Source: CAD feature listing. Evaluate the final solid. Frame: model axes, mm. A direction names the side the tool comes from. Round coordinates to 2 decimals unless told otherwise and drop trailing zeros. Write each loop counter-clockwise with the first axis right and the second up, starting at its lowest first coordinate (ties: lowest second). Pieces come first, ordered by that corner, then holes. Notation, with made-up numbers: M 72,-12 L 90,-12 A29 ccw 90,26 Z; hole C 83,-18 d5. An arc over 180 degrees is marked long. Answer in a Markdown table with one row per item. Add a question column.
Item 1: Set-up query: faces 1 (the face through (13.037, 7.419, 3.479)), 2 (the face through (-11.9, 6.97, 0.79)), 3 (the face through (-11.9, 6.97, 6.21)). Return all of +Z, -Z, +X, -X, +Y, -Y with unobstructed straight access to the full face (end or side cutting, diameter ignored); none if empty.
Item 2: Material intervals for probe 1 along Y at (x, z) = (0, 3.25); probe 2 along X at (y, z) = (-9, 5); probe 3 along X at (y, z) = (-23.5, 1), sorted ascending.
Item 3: Contact query for flat-ended pins moving along their axis: pin 1 (13 mm diameter, centred on x = 0, y = 0, fed in from +Z); pin 2 (3 mm diameter, centred on x = 27, z = 4.5, fed in from -Y); pin 3 (10 mm diameter, centred on x = -18.5, y = 7, fed in from -Z); pin 4 (3 mm diameter, centred on x = -28.5, z = 1.5, fed in from +Y). Output: stop coordinate, or through.
Item 4: Cut plane B-B on z = 4. Give the number of separate pieces and of enclosed holes in the cut face, and give its area (3 significant figures).
Item 5: Cut plane A-A on x = 0. Return loops of the section in (y, z), and give its area (3 significant figures).
Item 6: Mould query, pull axis Y, two halves, no side actions, for faces 4 (the face through (-8.69, -6.66, 3.45)), 5 (the face through (0, -14, 6)), 6 (the face through (35.38, -20.96, 6.87)). Classes: released by +Y, released by -Y, zero draft, split by the parting line, or undercut.
from build123d import *

# Parameters (mm, degrees)
F0_R     = 10.95
F1_DEPTH = 7
F2_R     = 2
F3_SIZE  = 2


with BuildPart() as f1:
    # F0 (on Top) → F1 (new body)
    with BuildSketch(Plane.XY):
        with BuildLine():
            ThreePointArc((14.816938, -2.33631), (12.990381, 7.5), (5.385165, 14))
            ThreePointArc((5.385165, 14), (0, 43), (-5.385165, 14))
            ThreePointArc((-5.385165, 14), (-12.990381, 7.5), (-14.816938, -2.33631))
            ThreePointArc((-14.816938, -2.33631), (-37.239092, -21.5), (-9.431773, -11.66369))
            ThreePointArc((-9.431773, -11.66369), (0, -15), (9.431773, -11.66369))
            ThreePointArc((9.431773, -11.66369), (37.239092, -21.5), (14.816938, -2.33631))
        make_face()
        with Locations((-24.248711, -14)):
            Circle(F0_R, mode=Mode.SUBTRACT)
        with Locations((24.248711, -14)):
            Circle(F0_R, mode=Mode.SUBTRACT)
        Circle(F0_R, mode=Mode.SUBTRACT)
        with Locations((0, 28)):
            Circle(F0_R, mode=Mode.SUBTRACT)
    extrude(amount=F1_DEPTH)

    # F2
    f2_edges = [f1.edges().sort_by_distance(p)[0] for p in [
        (-9.431773, -11.66369, 3.5),
        (9.431773, -11.66369, 3.5),
        (14.816938, -2.33631, 3.5),
        (5.385165, 14, 3.5),
        (-5.385165, 14, 3.5),
        (-14.816938, -2.33631, 3.5),
    ]]
    fillet(f2_edges, radius=F2_R)

    # F3
    f3_edges = [f1.edges().sort_by_distance(p)[0] for p in [
        (37.239092, -21.5, 0),
        (37.239092, -21.5, 7),
    ]]
    chamfer(f3_edges, length=F3_SIZE)


solid = f1.part
Results below:
| question | item | result |
|---|---|---|
| 1 | face 1 | +Z, -Z, +X |
| 1 | face 2 | -Z, -X |
| 1 | face 3 | +Z, -X |
| 2 | probe 1 | -15 to -10.95, 10.95 to 17.05, 38.95 to 43 |
| 2 | probe 2 | -38.39 to -33.99, -14.51 to -6.24, 6.24 to 14.51, 33.99 to 38.39 |
| 2 | probe 3 | -34.53 to -29.69, -18.8 to -13.97, 13.97 to 18.8, 29.69 to 34.53 |
| 3 | pin 1 | through |
| 3 | pin 2 | y = -28.95 |
| 3 | pin 3 | z = 1.78 |
| 3 | pin 4 | y = 0.73 |
| 4 | separate pieces | 1 |
| 4 | enclosed holes | 4 |
| 4 | area | 1,290 mm2 |
| 5 | outline | M -15,2 L -13,0 L -10.95,0 L -10.95,7 L -13,7 L -15,5 Z; M 10.95,0 L 17.05,0 L 17.05,7 L 10.95,7 Z; M 38.95,0 L 41,0 L 43,2 L 43,5 L 41,7 L 38.95,7 Z |
| 5 | area | 91.4 mm2 |
| 6 | face 4 | undercut |
| 6 | face 5 | released by -Y |
| 6 | face 6 | split by the parting line |
